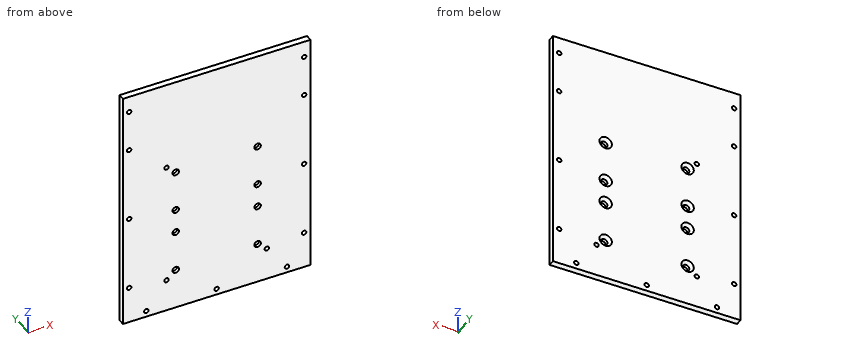
from build123d import *

# Parameters (mm, degrees)
SKETCH1_W                                    = 189.992
SKETCH1_H                                    = 254
BOSS_EXTRUDE1_DEPTH                          = 6.35
SKETCH3_R                                    = 2.2479
CUT_EXTRUDE1_DEPTH                           = 7.35
SKETCH4_R                                    = 2.2479
CUT_EXTRUDE2_DEPTH                           = 7.35
CSK_FOR_M6_COUNTERSUNK_FLAT_HEAD_SCR_2_COUNT = 2
CSK_FOR_M6_COUNTERSUNK_FLAT_HEAD_SCR_2_PITCH = 42.5196
CSK_FOR_M6_COUNTERSUNK_FLAT_HEAD_SCR_3_COUNT = 2
CSK_FOR_M6_COUNTERSUNK_FLAT_HEAD_SCR_3_PITCH = 24.9936
CSK_FOR_M6_COUNTERSUNK_FLAT_HEAD_SCR_4_COUNT = 2
CSK_FOR_M6_COUNTERSUNK_FLAT_HEAD_SCR_4_PITCH = 67.5132


with BuildPart() as part:
    # Sketch1 → Boss-Extrude1 (new body)
    with BuildSketch(Plane(origin=(0, 0, 0), x_dir=(1, 0, 0), z_dir=(0, 1, 0))):
        Rectangle(SKETCH1_W, SKETCH1_H)
    extrude(amount=BOSS_EXTRUDE1_DEPTH)

    # Sketch3 → Cut-Extrude1 (cut, through all)
    with BuildSketch(Plane(origin=(0, 6.35, 0), x_dir=(1, 0, 0), z_dir=(0, 1, 0))):
        with Locations((-88.646, -109.9312)):
            Circle(SKETCH3_R)
        with Locations((-88.646, -66.9544)):
            Circle(SKETCH3_R)
        with Locations((-88.646, 10.7442)):
            Circle(SKETCH3_R)
        with Locations((-88.646, 88.4428)):
            Circle(SKETCH3_R)
        with Locations((-50.8, 93.1164)):
            Circle(SKETCH3_R)
        with Locations((-71.247, 120.65)):
            Circle(SKETCH3_R)
        with Locations((0, 120.65)):
            Circle(SKETCH3_R)
    cut_extrude1 = extrude(amount=-CUT_EXTRUDE1_DEPTH, mode=Mode.SUBTRACT)

    # Mirror1: Cut-Extrude1 across plane
    add(cut_extrude1.mirror(Plane(origin=(0, 0, 0), x_dir=(0, 0, 1), z_dir=(1, 0, 0))), mode=Mode.SUBTRACT)

    # Sketch4 → Cut-Extrude2 (cut, through all)
    with BuildSketch(Plane(origin=(0, 6.35, 0), x_dir=(1, 0, 0), z_dir=(0, 1, 0))):
        with Locations((-50.8, -33.8836)):
            Circle(SKETCH4_R)
    extrude(amount=-CUT_EXTRUDE2_DEPTH, mode=Mode.SUBTRACT)

    # Sketch7 → CSK for M6 Countersunk Flat Head Screw1 (revolve, cut)
    with BuildSketch(Plane(origin=(-41.5036, 6.35, -17.145), x_dir=(0, 0, 1), z_dir=(1, 0, 0))):
        Polygon((0, 0), (0, 46.984041764), (3.302, 45), (3.302, 2.9972), (6.2992, 0), align=None)
    csk_for_m6_countersunk_flat_head_screw1 = revolve(axis=Axis((-41.5036, 12.7, -17.145), (0, -1, 0)), mode=Mode.SUBTRACT)

    # CSK for M6 Countersunk Flat Head Scr 2: CSK for M6 Countersunk Flat Head Screw1 ×2
    with Locations(*[(0, 0, i * CSK_FOR_M6_COUNTERSUNK_FLAT_HEAD_SCR_2_PITCH) for i in range(1, CSK_FOR_M6_COUNTERSUNK_FLAT_HEAD_SCR_2_COUNT)]):
        add(csk_for_m6_countersunk_flat_head_screw1, mode=Mode.SUBTRACT)

    # CSK for M6 Countersunk Flat Head Scr 3: CSK for M6 Countersunk Flat Head Screw1 ×2
    with Locations(*[(0, 0, -i * CSK_FOR_M6_COUNTERSUNK_FLAT_HEAD_SCR_3_PITCH) for i in range(1, CSK_FOR_M6_COUNTERSUNK_FLAT_HEAD_SCR_3_COUNT)]):
        add(csk_for_m6_countersunk_flat_head_screw1, mode=Mode.SUBTRACT)

    # CSK for M6 Countersunk Flat Head Scr 4: CSK for M6 Countersunk Flat Head Screw1 ×2
    with Locations(*[(0, 0, -i * CSK_FOR_M6_COUNTERSUNK_FLAT_HEAD_SCR_4_PITCH) for i in range(1, CSK_FOR_M6_COUNTERSUNK_FLAT_HEAD_SCR_4_COUNT)]):
        add(csk_for_m6_countersunk_flat_head_screw1, mode=Mode.SUBTRACT)

    # Mirror2: CSK for M6 Countersunk Flat Head Screw1 across plane
    add(csk_for_m6_countersunk_flat_head_screw1.mirror(Plane(origin=(0, 0, 0), x_dir=(0, 0, 1), z_dir=(1, 0, 0))), mode=Mode.SUBTRACT)

    # Mirror2 copy 1 sketch → Mirror2 copy 1 (revolve, cut)
    with BuildSketch(Plane(origin=(41.5036, 6.35, 25.3746), x_dir=(0, 0, 1), z_dir=(-1, 0, 0))):
        Polygon((0, 0), (0, -46.984041764), (3.302, -45), (3.302, -2.9972), (6.2992, 0), align=None)
    revolve(axis=Axis((41.5036, 12.7, 25.3746), (0, 1, 0)), mode=Mode.SUBTRACT)

    # Mirror2 copy 2 sketch → Mirror2 copy 2 (revolve, cut)
    with BuildSketch(Plane(origin=(41.5036, 6.35, -42.1386), x_dir=(0, 0, 1), z_dir=(-1, 0, 0))):
        Polygon((0, 0), (0, -46.984041764), (3.302, -45), (3.302, -2.9972), (6.2992, 0), align=None)
    revolve(axis=Axis((41.5036, 12.7, -42.1386), (0, 1, 0)), mode=Mode.SUBTRACT)

    # Mirror2 copy 3 sketch → Mirror2 copy 3 (revolve, cut)
    with BuildSketch(Plane(origin=(41.5036, 6.35, -84.6582), x_dir=(0, 0, 1), z_dir=(-1, 0, 0))):
        Polygon((0, 0), (0, -46.984041764), (3.302, -45), (3.302, -2.9972), (6.2992, 0), align=None)
    revolve(axis=Axis((41.5036, 12.7, -84.6582), (0, 1, 0)), mode=Mode.SUBTRACT)


solid = part.part
Read the model definition and answer for the solid it produces. Units are mm, in the model's axes. Coordinates: 2 decimals unless noted, no trailing zeros. Use one line per item in the form item = value.
(1) Given pin 1 Ø10.5 at (x, z) = (41.5, -42.14) entering from +Y; pin 2 Ø8.5 at (x, z) = (41.5, 25.37) entering from +Y, each flat-ended and moving along its own axis, determine where each tip first touches the part or whether it passes through.
Computed values:
pin_1 = 5.3
pin_2 = 4.31
(2) Straight lines are drawn through the part: L1, parallel to X at y = 2.5, z = -120.65; L2, parallel to Z at x = -50.5, y = 3.25; L3, parallel to X at y = 1.5, z = -17.5. For each, find the intervals that lie inside material, in ascending order.
Computed values:
L1 = -95 to -73.49, -69 to -2.25, 2.25 to 69, 73.49 to 95
L2 = -127 to -95.34, -90.89 to 31.66, 36.11 to 127
L3 = -95 to -44.79, -38.22 to 38.22, 44.79 to 95
(3) Section A-A, the plane y = 5 is taken. Give the number of separate pieces and of enclosed holes in the cut face, then the cut area to 3 significant figures.
Computed values:
separate_pieces = 1
enclosed_holes = 22
area = 47,400 mm²
